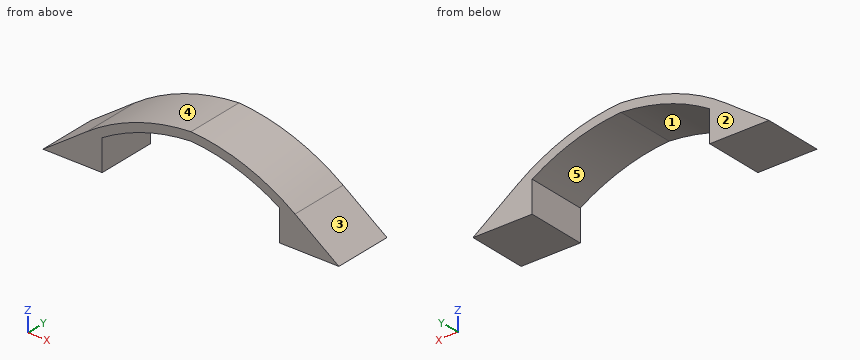
```python
from build123d import *

# Parameters (mm, degrees)
F1_DEPTH = 22.225


with BuildPart() as f1:
    # F0 (on Front) → F1 (new body)
    with BuildSketch(Plane.XZ):
        with BuildLine():
            Line((-39.084297, 11.671778), (-55.5625, 0))
            Line((-55.5625, 0), (-33.3375, 0))
            Line((-33.3375, 0), (-33.3375, 11.671778))
            ThreePointArc((-33.3375, 11.671778), (-17.317547, 18.99793), (0, 22.225))
            ThreePointArc((0, 22.225), (17.317547, 18.99793), (33.3375, 11.671778))
            Line((33.3375, 11.671778), (33.3375, 0))
            Line((33.3375, 0), (55.5625, 0))
            Line((55.5625, 0), (39.084297, 11.671778))
            ThreePointArc((39.084297, 11.671778), (20.504205, 21.274866), (0, 25.4))
            ThreePointArc((0, 25.4), (-20.504205, 21.274866), (-39.084297, 11.671778))
        make_face()
    extrude(amount=F1_DEPTH)


solid = f1.part
```
The listing builds one solid part. Answer for the finished solid, in the listing's coordinates (mm). Face numbers are marked on the shaded views. A direction names the side the tool comes from. Give positions to 0.01 mm unless a question says otherwise; leave off trailing zeros. Loops run counter-clockwise (first coordinate to the right, second up) from the corner with the lowest first, then second, coordinate; pieces in that order, holes last. Notation, with made-up numbers: M 74.25,-21.75 L 80.25,-21.75 A29 ccw 80.25,17.25 Z; hole C 41.25,66.5 d3. An arc over 180 degrees is marked long. One line per item, written item: value.
1. Section C-C on z = 14.5 is taken. Determine the outline of the cut face in (x, y) (3 decimals), plus the area to 3 significant figures.
Found:
outline: M -34.788,-22.225 L -28.296,-22.225 L -28.296,0 L -34.788,0 Z; M 28.296,-22.225 L 34.788,-22.225 L 34.788,0 L 28.296,0 Z
area: 289 mm^2
2. For the marked faces 4 and 5, determine the directions among +Z, -Z, +X, -X, +Y, -Y from which every point of the face is accessible in a straight line to the end or side of a thin tool.
Found:
face 4: +Z, -X, +Y, -Y
face 5: -Z, +Y, -Y
3. Section A-A on z = 21 is taken. Determine the outline of the cut face in (x, y) (3 decimals).
Found:
outline: M -21.273,-22.225 L -9.497,-22.225 L -9.497,0 L -21.273,0 Z; M 9.497,-22.225 L 21.273,-22.225 L 21.273,0 L 9.497,0 Z
4. Section D-D on x = 20.5 is taken. Determine the outline of the cut face in (y, z) (3 decimals).
Found:
outline: M -22.225,17.908 L 0,17.908 L 0,21.276 L -22.225,21.276 Z
5. Find the intervals of material crossed by probe 1 along X at (y, z) = (-14.75, 12); probe 2 along X at (y, z) = (-18, 11); probe 3 along Z at (x, y) = (-18.5, -6), in increasing order.
Found:
probe 1: -38.62 to -32.8, 32.8 to 38.62
probe 2: -40.03 to -33.34, 33.34 to 40.03
probe 3: 18.61 to 21.95
6. For a pull along X with two mould halves and no side action, classify the marked faces 1, 2 and 3 as pulls with the +X half, pulls with the -X half, needs draft (parallel to the pull), parting line crosses it, or undercut.
Found:
face 1: undercut
face 2: needs draft
face 3: pulls with the +X half
7. Each of these flat-tipped pins is pushed along its axis until it touches: P1, Ø1, axis at x = -8, y = -17.5, coming from the -Z side; P2, Ø2, axis at x = 32.5, y = -8.5, coming from the +Z side; P3, Ø12, axis at y = -7, z = 11, coming from the +X side. Where does it stop, or does it pass through?
Found:
P1: z = 21.19
P2: z = 16.39
P3: x = 48.5
8. Section B-B on y = -18 is taken. Determine the outline of the cut face in (x, z) (1 decimal).
Found:
outline: M -55.6,0 L -33.3,0 L -33.3,11.7 A72.2 cw 0,22.2 A72.2 cw 33.3,11.7 L 33.3,0 L 55.6,0 L 39.1,11.7 A75.3 ccw 0,25.4 A75.3 ccw -39.1,11.7 Z
